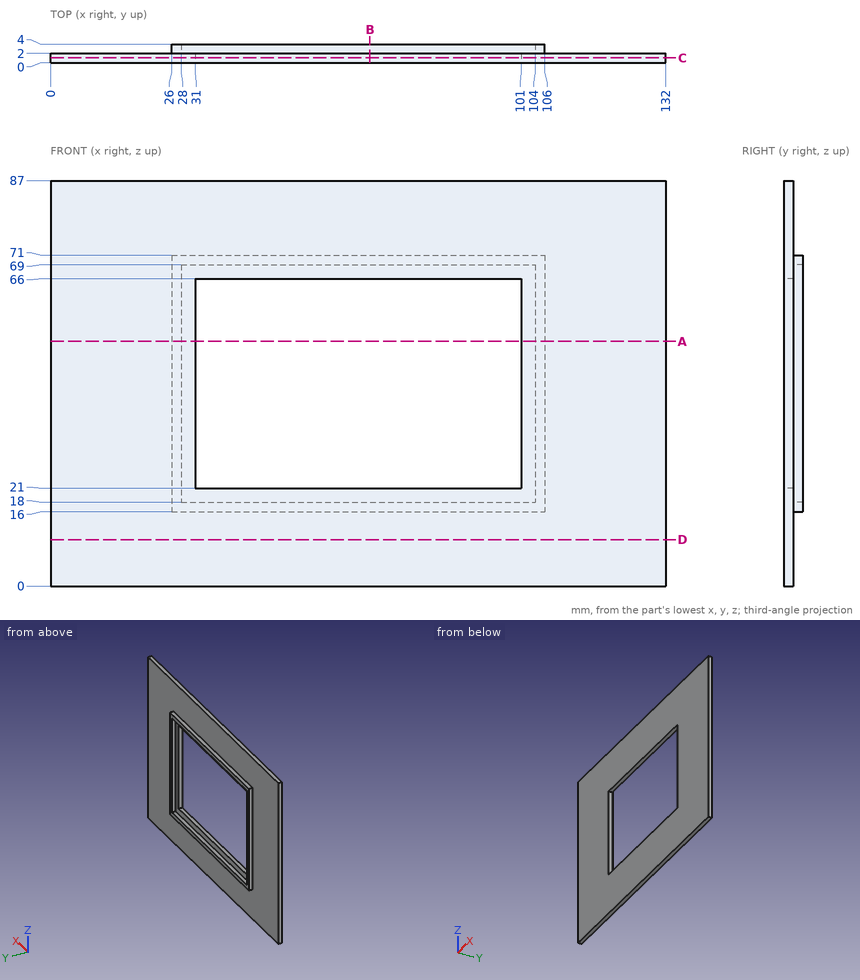
Here's the drawing with two shaded views (mm, measured from the low corner). I have some questions. Coordinates: 2 decimals unless noted, no trailing zeros. Write each loop counter-clockwise with the first axis right and the second up, starting at its lowest first coordinate (ties: lowest second). Pieces come first, ordered by that corner, then holes. Notation, with made-up numbers: (28.25, 20.5) -> (35.25, 20.5) arc R23 cw to (35.25, 44.5) -> close; hole circle Ø7 at (51, 12). An arc over 180 degrees is marked (long way). One line per question, with ' | ' between items. Start each with the question number.
1. Please list where these lines run through material, in increasing order: line 1 along X through (y, z) = (2.25, 39); line 2 along Z through (x, y) = (80.5, 1.35); line 3 along Z through (x, y) = (89, 3.1).
2. If we section it at D-D (z = 10): Please give me the cut outline in (x, y).
3. If we section it at B-B (x = 68.5): Please give me the cut outline in (y, z), and give its area (3 significant figures).
4. Will these pins go through, and if not, where does the flat tip stop? P1, Ø1.6, axis at y = 3, z = 41.5, coming from the -X side; P2, Ø0.6, axis at y = 3, z = 45.5, coming from the +X side.
5. If we section it at A-A (z = 52.5): Please give me the cut outline in (x, y), and give its area (3 significant figures).
6. If we section it at C-C (y = 1): Please give me the cut outline in (x, z).
Return value:
1) line 1: x = 26 to 28, 104 to 106 | line 2: z = 0 to 21, 66 to 87 | line 3: z = 16 to 18, 69 to 71
2) outline: (0, 0) -> (132, 0) -> (132, 2) -> (0, 2) -> close
3) outline: (0, 0) -> (2, 0) -> (2, 16) -> (4, 16) -> (4, 18) -> (2, 18) -> (2, 21) -> (0, 21) -> close; (0, 66) -> (2, 66) -> (2, 69) -> (4, 69) -> (4, 71) -> (2, 71) -> (2, 87) -> (0, 87) -> close | area: 92.0 mm²
4) P1: stops at x = 26 | P2: stops at x = 106
5) outline: (0, 0) -> (31, 0) -> (31, 2) -> (28, 2) -> (28, 4) -> (26, 4) -> (26, 2) -> (0, 2) -> close; (101, 0) -> (132, 0) -> (132, 2) -> (106, 2) -> (106, 4) -> (104, 4) -> (104, 2) -> (101, 2) -> close | area: 132 mm²
6) outline: (0, 0) -> (132, 0) -> (132, 87) -> (0, 87) -> close; hole (31, 21) -> (101, 21) -> (101, 66) -> (31, 66) -> close
